The listing builds one solid part. Answer for the finished solid, in the listing's coordinates (mm). A direction names the side the tool comes from. Round coordinates to 2 decimals unless told otherwise and drop trailing zeros. Loops run counter-clockwise (first coordinate to the right, second up) from the corner with the lowest first, then second, coordinate; pieces in that order, holes last. Notation, with made-up numbers: M 14.25,-33.5 L 20.25,-33.5 A14 cw 20.25,-9.5 Z; hole C 34,63.25 d8. An arc over 180 degrees is marked long. Answer as a JSON object with one key per item and string values.
```python
from build123d import *

# Parameters (mm, degrees)
F0_W     = 70
F0_H     = 30
F1_DEPTH = 80
F2_R     = 5
F3_DEPTH = 50
F5_DEPTH = 10


with BuildPart() as f1:
    # F0 (on Top) → F1 (new body)
    with BuildSketch(Plane.XY):
        Rectangle(F0_W, F0_H)
    extrude(amount=F1_DEPTH)

    # F2 (on face) → F3 (join)
    with BuildSketch(Plane.XY.offset(80)):
        with Locations((-13.248, 0)):
            Circle(F2_R)
        with Locations((18.53054, 0)):
            Circle(F2_R)
    extrude(amount=F3_DEPTH)

    # F4 (on face) → F5 (cut)
    with BuildSketch(Plane.XZ.offset(15)):
        Polygon((8.690138, 62.054458), (25.116485, 59.377786), (19.221377, 74.941756), align=None)
        Polygon((-2.943005, 46.873943), (-11.033713, 75.867229), (-32.097282, 54.363828), align=None)
        Polygon((-25.11046, 2.536608), (-2.81477, 21.49697), (-30.38277, 31.325422), align=None)
        Polygon((33.337645, 25.32119), (16.663238, 44.953783), (7.998117, 20.697027), align=None)
    extrude(amount=-F5_DEPTH, mode=Mode.SUBTRACT)


solid = f1.part
```
Item 1: Which of the six approach directions +Z, -Z, +X, -X, +Y, -Y give full straight-line access (tool end or side, diameter ignored) to faces 1 (the face through (0, 15, 39)), 2 (the face through (-6.932, -10.07, 61.168)), 3 (the face through (13.535, 0.22, 104.65))?
Values follow:
{"face 1": "+Z, -Z, +X, -X, +Y", "face 2": "-Y", "face 3": "+Z"}
Item 2: The part is cut by section A-A (y = -6.5). Give the vertices of the cut face in (x, z).
Values follow:
{"outline": "M -35,0 L 35,0 L 35,80 L -35,80 Z; hole M -32.1,54.36 L -2.94,46.87 L -11.03,75.87 Z; hole M -30.38,31.33 L -25.11,2.54 L -2.81,21.5 Z; hole M 8,20.7 L 33.34,25.32 L 16.66,44.95 Z; hole M 8.69,62.05 L 25.12,59.38 L 19.22,74.94 Z"}
Item 3: Straight lines are drawn through the part: line 1 (Z direction, x = -13, y = -6.75); line 2 (X direction, y = -12, z = 66); line 3 (Z direction, x = -10.5, y = 12.5). For each, find the intervals that lie inside material, in ascending order.
Values follow:
{"line 1": "0 to 12.84, 25.13 to 49.46, 73.86 to 80", "line 2": "-35 to -20.7, -8.28 to 11.91, 22.61 to 35", "line 3": "0 to 80"}
Item 4: The part is cut by section C-C (z = 12). Give the vertices of the cut face in (x, y).
Values follow:
{"outline": "M -35,-15 L -26.84,-15 L -26.84,-5 L -13.98,-5 L -13.98,-15 L 35,-15 L 35,15 L -35,15 Z"}
Item 5: The part is cut by section D-D (y = 0). Give the vertices of the cut face in (x, z).
Values follow:
{"outline": "M -35,0 L 35,0 L 35,80 L 23.53,80 L 23.53,130 L 13.53,130 L 13.53,80 L -8.25,80 L -8.25,130 L -18.25,130 L -18.25,80 L -35,80 Z"}
Item 6: Flat-ended cylindrical pins translate along their axes: P1, Ø1.5, axis at x = -7, y = -1, coming from the +Z side; P2, Ø3, axis at y = 2.5, z = 103.5, coming from the -X side. Find the tip coordinate at first contact, or state that the pin passes through.
Values follow:
{"P1": "z = 80", "P2": "x = -18.15"}
Item 7: The part is cut by section B-B (z = 88.5). Give the vertices of the cut face in (x, y).
Values follow:
{"outline": "C -13.25,0 d10; C 18.53,0 d10"}
Item 8: Determine the mould class of faces 4 (the face through (35, 0, 39)), 5 (the face through (18, 0, 130)), 6 (the face through (16.788, -10.07, 60.735)), 7 (the face through (-17.72, -10.07, 50.67)) for opening direction Z: released by +Z, released by -Z, zero draft, split by the parting line, or undercut.
Values follow:
{"face 4": "zero draft", "face 5": "released by +Z", "face 6": "undercut", "face 7": "undercut"}
